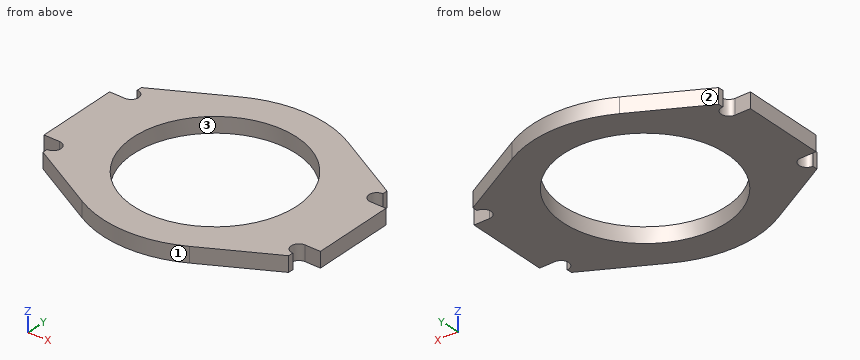
Autodesk Inventor part; units mm, degrees
ref_plane "YZ Plane" through (0, 0, 0) normal (1, 0, 0) x (0, 1, 0)
ref_plane "XZ Plane" through (0, 0, 0) normal (0, 1, 0) x (-1, 0, 0)
ref_plane "XY Plane" through (0, 0, 0) normal (0, 0, 1) x (1, 0, 0)
sketch "スケッチ1" plane through (0, 0, 0) normal (0, 0, 1) x (1, 0, 0)
  circle A0 centre (0, 0) radius 16
  circle A1 centre (0, 0) radius 22
  dimension "d0" = 32
  dimension "d7" = 6
extrude "押し出し1" add sketch "スケッチ1" along normal blind 3
sketch "スケッチ2" plane through (0, 0, 0) normal (0, 0, -1) x (-1, 0, 0)
  line L0 (-27, 8) -> (-27, -8)
  line L1 (27, -8) -> (27, 8)
  line L2 (24, -8) -> (27, -8)
  line L3 (-27, -8) -> (-24, -8)
  line L4 (-24, 8) -> (-27, 8)
  line L5 (27, 8) -> (24, 8)
  line L6 (-24, 12) -> (-24, 11)
  line L7 (-24, -11) -> (-24, -12)
  line L8 (24, -12) -> (24, -11)
  line L9 (24, 11) -> (24, 12)
  line L10 (-24, -12) -> (-10.5005, -19.3323)
  line L11 (10.5005, -19.3323) -> (24, -12)
  line L12 (24, 12) -> (10.5005, 19.3323)
  line L13 (-10.5005, 19.3323) -> (-24, 12)
  circle A0 centre (0, 0) radius 22
  arc A1 (24, -8) -> (24, -11) centre (24, -9.5) ccw
  arc A2 (24, 11) -> (24, 8) centre (24, 9.5) ccw
  arc A3 (-24, 8) -> (-24, 11) centre (-24, 9.5) ccw
  arc A4 (-24, -11) -> (-24, -8) centre (-24, -9.5) ccw
  point P0 (-27, 0)
  point P1 (27, 0)
  dimension "d10" = 54
  dimension "d11" = 16
  dimension "d13" = 48
  dimension "d14" = 24
  dimension "d17" = 3
extrude "押し出し2" add sketch "スケッチ2" against normal blind 3 contours L4 A3 L6 L13 A0 L10 L7 A4 L3 L0 | L12 L9 A2 L5 L1 L2 A1 L8 L11 A0
properties part number "RS555-71K_MotorsupportPolica" material "ポリカーボネート、クリア"
For this review, take the finished solid that the model builds, in its own axes (mm). Face numbers are marked on the shaded views. Give positions to 0.01 mm unless a question says otherwise; leave off trailing zeros. Write each loop counter-clockwise with the first axis right and the second up, starting at its lowest first coordinate (ties: lowest second). Pieces come first, ordered by that corner, then holes. Notation, with made-up numbers: (38, -8.5) -> (74, -8.5) arc R19 cw to (74, 15.5) -> close; hole circle Ø7 at (47.5, 81). An arc over 180 degrees is marked (long way). Use CSV: the item, a comma, the result in double quotes.
Q1. Take a section at B-B, the plane x = 2. Write out the cut boundary in (y, z), then the cut area to 3 significant figures.
Conclusion:
outline,"(-21.91, 0) -> (-15.87, 0) -> (-15.87, 3) -> (-21.91, 3) -> close; (15.87, 0) -> (21.91, 0) -> (21.91, 3) -> (15.87, 3) -> close"
area,"36.2 mm2"
Q2. To check wall thickness, follow probe 1 along Y at (x, z) = (0, 2); probe 2 along X at (y, z) = (-3.5, 2.45); probe 3 along X at (y, z) = (6, 0.4). State the ranges of each line that lie inside material, in increasing order. Write a range as [from, to].
Conclusion:
probe 1,"[-22, -16], [16, 22]"
probe 2,"[-27, -15.61], [15.61, 27]"
probe 3,"[-27, -14.83], [14.83, 27]"
Q3. Take a section at D-D, the plane y = 18. Write out the cut boundary in (x, z).
Conclusion:
outline,"(-12.95, 0) -> (12.95, 0) -> (12.95, 3) -> (-12.95, 3) -> close"
Q4. Take a section at A-A, the plane y = 0. Write out the cut boundary in (x, z).
Conclusion:
outline,"(-27, 0) -> (-16, 0) -> (-16, 3) -> (-27, 3) -> close; (16, 0) -> (27, 0) -> (27, 3) -> (16, 3) -> close"
Q5. Mouldability with a two-part tool opening along Y and no side actions: class the marked faces 1, 2 and 3 as pulls with the +Y half, pulls with the -Y half, needs draft (parallel to the pull), parting line crosses it, or undercut.
Conclusion:
face 1,"pulls with the -Y half"
face 2,"pulls with the +Y half"
face 3,"undercut"
Q6. For P1, Ø0.8, axis at y = 11.5, z = 1, coming from the +X side; P2, Ø1.5, axis at x = 26, z = 1.5, coming from the -Y side; P3, Ø0.9, axis at x = -25.5, z = 2, coming from the +Y side; P4, Ø2, axis at x = 6, y = 12, coming from the -Z side, all flat-tipped, find the tip position at first contact; note any pin that passes through.
Conclusion:
P1,"x = 24"
P2,"y = -8"
P3,"y = 8"
P4,"through"
Q7. Take a section at C-C, the plane z = 0.85. Write out the cut boundary in (x, y), then the cut area to 3 significant figures.
Conclusion:
outline,"(-27, -8) -> (-24, -8) arc R1.5 cw to (-24, -11) -> (-24, -12) -> (-10.5, -19.33) arc R22 ccw to (10.5, -19.33) -> (24, -12) -> (24, -11) arc R1.5 cw to (24, -8) -> (27, -8) -> (27, 8) -> (24, 8) arc R1.5 cw to (24, 11) -> (24, 12) -> (10.5, 19.33) arc R22 ccw to (-10.5, 19.33) -> (-24, 12) -> (-24, 11) arc R1.5 cw to (-24, 8) -> (-27, 8) -> close; hole circle Ø32 at (0, 0)"
area,"1,010 mm2"
